Autodesk Inventor part; units mm, degrees
ref_plane "YZ Plane" through (0, 0, 0) normal (1, 0, 0) x (0, 1, 0)
ref_plane "XZ Plane" through (0, 0, 0) normal (0, 1, 0) x (-1, 0, 0)
ref_plane "XY Plane" through (0, 0, 0) normal (0, 0, 1) x (1, 0, 0)
sketch "Sketch2" plane through (0, 0, 0) normal (0, 0, 1) x (1, 0, 0)
  line L0 (0, 264) -> (0, -44)
  line L1 (-160, 0) -> (960, 0)
  line L2 (0, 0) -> (205, 0)
  line L3 (800, 220) -> (0, 220)
  line L4 (0, 220) -> (0, 0)
  line L5 (800, 104.9146) -> (800, 220)
  line L6 (205, 0) -> (800, 104.9146)
  dimension "d7" = 220
  dimension "d20" = 800
  dimension "d34" = 10
  dimension "d37" = 205
extrude "Extrusion2" add sketch "Sketch2" along normal blind 15
sketch "Sketch5" plane through (0, 0, 0) normal (0, 0, -1) x (-1, 0, 0)
  line L0 (-800, 104.9146) -> (-800, 220)
  line L1 (-205, 0) -> (-800, 104.9146)
  line L2 (-800, 220) -> (-964, 220)
  line L3 (-964, 220) -> (-964, 133.8322)
  line L4 (-800, 104.9146) -> (-964, 133.8322)
  line L5 (0, 220) -> (0, 0)
  dimension "d40" = 964
extrude "Extrusion4" add sketch "Sketch5" against normal up to surface (15 mm away)
sketch "Sketch3" plane through (0, 0, 0) normal (0, 0, -1) x (-1, 0, 0)
  line L0 (0, 220) -> (0, 0)
  line L1 (-800, 220) -> (0, 220)
  line L2 (-800, 104.9146) -> (-800, 220)
  line L3 (-595, 220) -> (-595, 240)
  circle A0 centre (-695, 288) radius 22.4
  circle A1 centre (-889, 301) radius 19.15
  arc A2 (-851.1955, 340.9477) -> (-942.6088, 313.2921) centre (-889, 301) ccw
  arc A3 (-643.9036, 319.4509) -> (-731.2075, 335.8437) centre (-695, 288) ccw
  line L4 (-595, 240) -> (-643.9036, 319.4509)
  line L5 (-942.6088, 313.2921) -> (-964, 220)
  line L6 (-964, 220) -> (-595, 220)
  line L7 (-731.2075, 335.8437) -> (-767.8616, 308.1042)
  line L8 (-851.1955, 340.9477) -> (-819.4942, 310.9471)
  arc A4 (-819.4942, 310.9471) -> (-767.8616, 308.1042) centre (-792, 340) ccw
  dimension "d23" = 44.8
  dimension "d26" = 695
  dimension "d28" = 68
  dimension "d29" = 20
  dimension "d35" = 100
  dimension "d41" = 38.3
  dimension "d42" = 81
  dimension "d43" = 194
  dimension "d45" = 110
  dimension "d46" = 60
  dimension "d47" = 97
  dimension "d48" = 40
  dimension "d49" = 120
extrude "Extrusion3" add sketch "Sketch3" against normal up to surface (15 mm away)
equation "\"d47\" = 0.5 * d43"
properties part number "Plate" material "EN10025 P6 2004 S690QL"
Source: CAD feature listing. Evaluate the final solid. Frame: model axes, mm. A direction names the side the tool comes from. Coordinates: 2 decimals unless noted, no trailing zeros. Loops run counter-clockwise (first coordinate to the right, second up) from the corner with the lowest first, then second, coordinate; pieces in that order, holes last. Notation, with made-up numbers: (45, -27.5) -> (55, -27.5) arc R18 ccw to (55, 1.5) -> close; hole circle Ø1 at (56, 2.5). An arc over 180 degrees is marked (long way). One line per item, written item: value. Start each with the question number.
Q1. Line query: line 1 along Y through (x, z) = (97, 3); line 2 along X through (y, z) = (278.5, 12.5); line 3 along Y through (x, z) = (889, 4.25). Output: solid intervals per line, ascending.
Q2. Section query D-D, the plane y = 87.5. Return the cut outline in (x, z), and give its area (3 significant figures).
Q3. Mould query, pull axis X, two halves, no side actions, for faces 3 (the face through (871.31, 293.67, 7.4)), 4 (the face through (953.155, 267.299, 7.395)), 5 (the face through (674.31, 279.42, 7.4)), 6 (the face through (619.11, 279.17, 7.4)). Classes: pulls with the +X half, pulls with the -X half, needs draft (parallel to the pull), parting line crosses it, or undercut.
Q4. Contact query for flat-ended pins moving along their axis: P1, Ø8, axis at x = 679.5, z = 12.5, coming from the -Y side; P2, Ø6, axis at y = 233, z = 11, coming from the +X side; P3, Ø2, axis at y = 233.5, z = 7, coming from the -X side. Output: stop coordinate, or through.
Q5. Section query B-B, the plane z = 11.25. Return the cut outline in (x, y).
Q6. Section query C-C, the plane x = 695. Return the cut outline in (y, z), and give its area (3 significant figures).
Q7. Section query A-A, the plane x = 889. Return the cut outline in (y, z).
Q8. Set-up query: faces 1 (the face through (489, 141, 15)), 2 (the face through (749.278, 322.168, 7.395)). Return all of +Z, -Z, +X, -X, +Y, -Y with unobstructed straight access to the full face (end or side cutting, diameter ignored); none if empty.
Results:
1. line 1: 0 to 220
1. line 2: 618.7 to 674.71, 715.29 to 950.59
1. line 3: 120.61 to 281.85, 320.15 to 356
2. outline: (0, 0) -> (701.24, 0) -> (701.24, 15) -> (0, 15) -> close
2. area: 10,500 mm^2
3. face 3: undercut
3. face 4: pulls with the +X half
3. face 5: undercut
3. face 6: pulls with the -X half
4. P1: y = 82.96
4. P2: x = 961.71
4. P3: x = 595
5. outline: (0, 0) -> (205, 0) -> (800, 104.91) -> (964, 133.83) -> (964, 220) -> (942.61, 313.29) arc R55 ccw to (851.2, 340.95) -> (819.49, 310.95) arc R40 cw to (767.86, 308.1) -> (731.21, 335.84) arc R60 ccw to (643.9, 319.45) -> (595, 240) -> (595, 220) -> (0, 220) -> close; hole circle Ø44.8 at (695, 288); hole circle Ø38.3 at (889, 301)
6. outline: (86.4, 0) -> (265.6, 0) -> (265.6, 15) -> (86.4, 15) -> close; (310.4, 0) -> (348, 0) -> (348, 15) -> (310.4, 15) -> close
6. area: 3,250 mm^2
7. outline: (120.61, 0) -> (281.85, 0) -> (281.85, 15) -> (120.61, 15) -> close; (320.15, 0) -> (356, 0) -> (356, 15) -> (320.15, 15) -> close
8. face 1: +Z, +X, -X, +Y, -Y
8. face 2: +Z, -Z, +Y
